Work out the finished part from the listing and answer in its coordinate system (mm). Face numbers are marked on the shaded views. A direction names the side the tool comes from. Coordinates: 2 decimals unless noted, no trailing zeros. Loops run counter-clockwise (first coordinate to the right, second up) from the corner with the lowest first, then second, coordinate; pieces in that order, holes last. Notation, with made-up numbers: (38.25, 76.25) -> (59.25, 76.25) arc R20 cw to (59.25, 97.25) -> close; hole circle Ø11 at (70.5, -3.75). An arc over 180 degrees is marked (long way). Use a Markdown table: item, result.
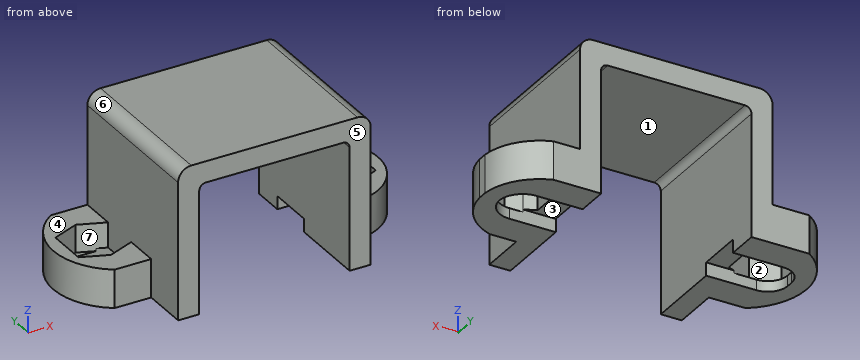
from build123d import *

# Parameters (mm, degrees)
EXTRUDE_1_DEPTH      = 11.4
SKETCH_2_W           = 11.4
SKETCH_2_H           = 8.3
CUT_EXTRUDE_1_DEPTH  = 9.8
CUT_EXTRUDE_2_DEPTH  = 10.6
CUT_EXTRUDE_3_DEPTH  = 0.8
CUT_EXTRUDE_4_DEPTH  = 8.5
CUT_EXTRUDE_5_DEPTH  = 0.8
CUT_EXTRUDE_6_DEPTH  = 2.1
CUT_EXTRUDE_7_DEPTH  = 0.2
CUT_EXTRUDE_8_DEPTH  = 1
CUT_EXTRUDE_9_DEPTH  = 8.5
CUT_EXTRUDE_10_DEPTH = 1.9
CUT_EXTRUDE_11_DEPTH = 0.2
EXTRUDE_2_DEPTH      = 3.5
FILLET_1_R           = 0.5
FILLET_2_R           = 1
FILLET_3_R           = 1.5


with BuildPart() as part:
    # 草图1 → 凸台-拉伸1 (new body)
    with BuildSketch(Plane.XY.offset(1.6)):
        with BuildLine():
            Line((-10.088816953, -2.4), (9.3, -2.4))
            ThreePointArc((9.3, -2.4), (11.373008704, -0.957826085), (12.3, 1.391198782))
            Line((12.3, 1.391198782), (12.3, 2.108801218))
            ThreePointArc((12.3, 2.108801218), (11.373008704, 4.457826085), (9.3, 5.9))
            Line((9.3, 5.9), (-10.088816953, 5.9))
            ThreePointArc((-10.088816953, 5.9), (-12.3, 1.75), (-10.088816953, -2.4))
        make_face()
        with BuildLine():
            Line((-7.8, 0), (-10.8, 0))
            Line((-10.8, 0), (-11.007, 0.0828))
            Line((-11.007, 0.0828), (-11.007, 2))
            ThreePointArc((-11.007, 2), (-10.567660172, 3.060660172), (-9.507, 3.5))
            Line((-9.507, 3.5), (-8.05, 3.5))
            Line((-8.05, 3.5), (-7.3, 3.2))
            Line((-7.3, 3.2), (-7.3, 0.2))
            Line((-7.3, 0.2), (-7.8, 0))
        make_face(mode=Mode.SUBTRACT)
        with BuildLine():
            Line((7.3, 0.4), (7.3, 3.1))
            Line((7.3, 3.1), (8.188888889, 3.5))
            Line((8.188888889, 3.5), (9.206872393, 3.5))
            ThreePointArc((9.206872393, 3.5), (10.461862433, 2.99034879), (11.006177815, 1.75))
            ThreePointArc((11.006177815, 1.75), (10.461862433, 0.50965121), (9.206872393, 0))
            Line((9.206872393, 0), (8.188888889, 0))
            Line((8.188888889, 0), (7.3, 0.4))
        make_face(mode=Mode.SUBTRACT)
    extrude(amount=-EXTRUDE_1_DEPTH)

    # 草图2 → 切除-拉伸1 (cut)
    with BuildSketch(Plane(origin=(0, 0, -9.8), x_dir=(-1, 0, 0), z_dir=(0, 0, -1))):
        with Locations((0, 1.75)):
            Rectangle(SKETCH_2_W, SKETCH_2_H)
    extrude(amount=-CUT_EXTRUDE_1_DEPTH, mode=Mode.SUBTRACT)

    # 草图3 → 切除-拉伸2 (cut)
    with BuildSketch(Plane.XY.offset(1.6)):
        Polygon((-7.8, 0), (-10.8, 0), (-9.3, -0.6), align=None)
    extrude(amount=-CUT_EXTRUDE_2_DEPTH, mode=Mode.SUBTRACT)

    # 草图4 → 切除-拉伸3 (cut)
    with BuildSketch(Plane(origin=(0, 0, -9.8), x_dir=(-1, 0, 0), z_dir=(0, 0, -1))):
        Polygon((11.007, 0.0828), (10.8, 0), (11.007, 0), align=None)
    extrude(amount=-CUT_EXTRUDE_3_DEPTH, mode=Mode.SUBTRACT)

    # 草图5 → 切除-拉伸4 (cut)
    with BuildSketch(Plane.XY.offset(1.6)):
        with BuildLine():
            Line((-9.507, 3.5), (-8.05, 3.5))
            Line((-8.05, 3.5), (-7.3, 3.2))
            Line((-7.3, 3.2), (-7.3, 5.9))
            Line((-7.3, 5.9), (-10.088816953, 5.9))
            ThreePointArc((-10.088816953, 5.9), (-12.3, 1.75), (-10.088816953, -2.4))
            Line((-10.088816953, -2.4), (-7.3, -2.4))
            Line((-7.3, -2.4), (-7.3, 0.2))
            Line((-7.3, 0.2), (-9.3, -0.6))
            Line((-9.3, -0.6), (-11.007, 0.0828))
            Line((-11.007, 0.0828), (-11.007, 2))
            ThreePointArc((-11.007, 2), (-10.567660172, 3.060660172), (-9.507, 3.5))
        make_face()
    extrude(amount=-CUT_EXTRUDE_4_DEPTH, mode=Mode.SUBTRACT)

    # 草图6 → 切除-拉伸5 (cut)
    with BuildSketch(Plane(origin=(0, 0, -9.8), x_dir=(-1, 0, 0), z_dir=(0, 0, -1))):
        Polygon((7.3, 3.2), (8.05, 3.5), (5.7, 3.5), (5.7, 0), (7.8, 0), (7.3, 0.2), align=None)
    extrude(amount=-CUT_EXTRUDE_5_DEPTH, mode=Mode.SUBTRACT)

    # 草图7 → 切除-拉伸6 (cut)
    with BuildSketch(Plane.XY.offset(-6.9)):
        with BuildLine():
            Line((-9.507, 3.5), (-8.05, 3.5))
            Line((-8.05, 3.5), (-9.3, 4))
            Line((-9.3, 4), (-11.3, 3.2))
            Line((-11.3, 3.2), (-11.3, 0.2))
            Line((-11.3, 0.2), (-11.007, 0.0828))
            Line((-11.007, 0.0828), (-11.007, 2))
            ThreePointArc((-11.007, 2), (-10.567660172, 3.060660172), (-9.507, 3.5))
        make_face()
    extrude(amount=-CUT_EXTRUDE_6_DEPTH, mode=Mode.SUBTRACT)

    # 草图8 → 切除-拉伸7 (cut)
    with BuildSketch(Plane(origin=(0, 0, -9), x_dir=(-1, 0, 0), z_dir=(0, 0, -1))):
        Polygon((7.3, 3.2), (8.05, 3.5), (5.7, 3.5), (5.7, 0), (7.8, 0), (7.3, 0.2), align=None)
    extrude(amount=-CUT_EXTRUDE_7_DEPTH, mode=Mode.SUBTRACT)

    # 草图9 → 切除-拉伸8 (cut)
    with BuildSketch(Plane(origin=(0, 0, -9.8), x_dir=(-1, 0, 0), z_dir=(0, 0, -1))):
        Polygon((-7.3, 0.4), (-8.188888889, 0), (-5.7, 0), (-5.7, 3.5), (-8.188888889, 3.5), (-7.3, 3.1), align=None)
    extrude(amount=-CUT_EXTRUDE_8_DEPTH, mode=Mode.SUBTRACT)

    # 草图10 → 切除-拉伸9 (cut)
    with BuildSketch(Plane.XY.offset(1.6)):
        with BuildLine():
            Line((9.206872393, 0), (8.188888889, 0))
            Line((8.188888889, 0), (7.3, 0.4))
            Line((7.3, 0.4), (7.3, -2.4))
            Line((7.3, -2.4), (9.3, -2.4))
            ThreePointArc((9.3, -2.4), (11.373008704, -0.957826085), (12.3, 1.391198782))
            Line((12.3, 1.391198782), (12.3, 2.108801218))
            ThreePointArc((12.3, 2.108801218), (11.373008704, 4.457826085), (9.3, 5.9))
            Line((9.3, 5.9), (7.3, 5.9))
            Line((7.3, 5.9), (7.3, 3.1))
            Line((7.3, 3.1), (8.188888889, 3.5))
            Line((8.188888889, 3.5), (9.206872393, 3.5))
            ThreePointArc((9.206872393, 3.5), (10.461862433, 2.99034879), (11.006177815, 1.75))
            ThreePointArc((11.006177815, 1.75), (10.461862433, 0.50965121), (9.206872393, 0))
        make_face()
    extrude(amount=-CUT_EXTRUDE_9_DEPTH, mode=Mode.SUBTRACT)

    # 草图11 → 切除-拉伸10 (cut)
    with BuildSketch(Plane.XY.offset(-6.9)):
        with BuildLine():
            Line((9.206872393, 0), (8.188888889, 0))
            Line((8.188888889, 0), (9.3, -0.5))
            Line((9.3, -0.5), (11.3, 0.3))
            Line((11.3, 0.3), (11.3, 3.2))
            Line((11.3, 3.2), (9.3, 4))
            Line((9.3, 4), (8.188888889, 3.5))
            Line((8.188888889, 3.5), (9.206872393, 3.5))
            ThreePointArc((9.206872393, 3.5), (10.461862433, 2.99034879), (11.006177815, 1.75))
            ThreePointArc((11.006177815, 1.75), (10.461862433, 0.50965121), (9.206872393, 0))
        make_face()
    extrude(amount=-CUT_EXTRUDE_10_DEPTH, mode=Mode.SUBTRACT)

    # 草图12 → 切除-拉伸11 (cut)
    with BuildSketch(Plane.XY.offset(-8.8)):
        with BuildLine():
            Line((9.206872393, 0), (8.188888889, 0))
            Line((8.188888889, 0), (9.3, -0.5))
            Line((9.3, -0.5), (11.3, 0.3))
            Line((11.3, 0.3), (11.3, 3.2))
            Line((11.3, 3.2), (9.3, 4))
            Line((9.3, 4), (8.188888889, 3.5))
            Line((8.188888889, 3.5), (9.206872393, 3.5))
            ThreePointArc((9.206872393, 3.5), (10.461862433, 2.99034879), (11.006177815, 1.75))
            ThreePointArc((11.006177815, 1.75), (10.461862433, 0.50965121), (9.206872393, 0))
        make_face()
    extrude(amount=-CUT_EXTRUDE_11_DEPTH, mode=Mode.SUBTRACT)

    # 草图13 → 凸台-拉伸2 (add)
    with BuildSketch(Plane.XZ.offset(2.4)):
        Polygon((-7.3, 1.6), (7.3, 1.6), (7.3, -9.8), (5.7, -9.8), (5.7, 0), (-5.7, 0), (-5.7, -9.8), (-7.3, -9.8), align=None)
    extrude(amount=EXTRUDE_2_DEPTH)

    # 圆角1
    fillet_1_edges = [part.edges().sort_by_distance(p)[0] for p in [
        (5.7, 0, 0),
        (-5.7, 0, 0),
    ]]
    fillet(fillet_1_edges, radius=FILLET_1_R)

    # 圆角2
    fillet_2_edges = [part.edges().sort_by_distance(p)[0] for p in [
        (-7.3, 0, 1.6),
        (7.3, 0, 1.6),
    ]]
    fillet(fillet_2_edges, radius=FILLET_2_R)

    # 圆角3
    # the kernel refuses this fillet: 1.5 mm, written as the material it adds along each edge
    with BuildSketch(Plane(origin=(-11.007, 0, -9.8), x_dir=(1.0, 7.597747752272154e-12, 0), z_dir=(0, 0, 1))) as fillet_3_piece_1:
        with BuildLine():
            CenterArc((FILLET_3_R, FILLET_3_R), FILLET_3_R, 180, 90)
            Line((0, FILLET_3_R), (0, 0))
            Line((0, 0), (FILLET_3_R, 0))
        make_face()
    extrude(amount=0.8)


solid = part.part
Q1. Section B-B on x = 7.75 is taken. Determine the outline of the cut face in (y, z), and give its area (3 significant figures).
Solved:
| item | result |
|---|---|
| outline | (-2.4, -9.8) -> (0, -9.8) -> (0, -8.8) -> (0.2, -8.8) -> (0.2, -6.9) -> (-2.4, -6.9) -> close; (3.3, -8.8) -> (3.5, -8.8) -> (3.5, -9.8) -> (5.9, -9.8) -> (5.9, -6.9) -> (3.3, -6.9) -> close |
| area | 14.7 mm² |
Q2. Section C-C on y = -4.75 is taken. Determine the outline of the cut face in (x, z).
Solved:
| item | result |
|---|---|
| outline | (-7.3, -9.8) -> (-5.7, -9.8) -> (-5.7, -0.5) arc R0.5 cw to (-5.2, 0) -> (5.2, 0) arc R0.5 cw to (5.7, -0.5) -> (5.7, -9.8) -> (7.3, -9.8) -> (7.3, 0.6) arc R1 ccw to (6.3, 1.6) -> (-6.3, 1.6) arc R1 ccw to (-7.3, 0.6) -> close |
Q3. Section D-D on y = 0.75 is taken. Determine the outline of the cut face in (x, z).
Solved:
| item | result |
|---|---|
| outline | (-12.2, -9.8) -> (-10.81, -9.8) -> (-10.81, -9) -> (-11.3, -9) -> (-11.3, -6.9) -> (-12.2, -6.9) -> close; (-7.3, -8.8) -> (-5.7, -8.8) -> (-5.7, -0.5) arc R0.5 cw to (-5.2, 0) -> (5.2, 0) arc R0.5 cw to (5.7, -0.5) -> (5.7, -8.8) -> (7.3, -8.8) -> (7.3, 0.6) arc R1 ccw to (6.3, 1.6) -> (-6.3, 1.6) arc R1 ccw to (-7.3, 0.6) -> close; (10.67, -9.8) -> (12.2, -9.8) -> (12.2, -6.9) -> (11.3, -6.9) -> (11.3, -9) -> (10.67, -9) -> close |
Q4. Determine the mould class of the marked faces 5, 6 and 7 for opening direction Y: pulls with the +Y half, pulls with the -Y half, needs draft (parallel to the pull), parting line crosses it, or undercut.
Solved:
| item | result |
|---|---|
| face 5 | pulls with the -Y half |
| face 6 | needs draft |
| face 7 | undercut |
Q5. For the marked faces 1, 2, 3 and 4, determine the directions among +Z, -Z, +X, -X, +Y, -Y from which every point of the face is accessible in a straight line to the end or side of a thin tool.
Solved:
| item | result |
|---|---|
| face 1 | -Z, +Y, -Y |
| face 2 | +Z |
| face 3 | -Z |
| face 4 | +Z, -X, +Y, -Y |
Q6. Section A-A on z = -2.5 is taken. Determine the outline of the cut face in (x, y).
Solved:
| item | result |
|---|---|
| outline | (-7.3, -5.9) -> (-5.7, -5.9) -> (-5.7, 5.9) -> (-7.3, 5.9) -> close; (5.7, -5.9) -> (7.3, -5.9) -> (7.3, 5.9) -> (5.7, 5.9) -> close |
Q7. Consider line 1 (X direction, y = -4.25, z = -2.5); line 2 (Z direction, x = -3.5, y = -3); line 3 (X direction, y = 3, z = -8.25). Determine where each line is inside the solid, lowest interval first. Write a range as [from, to].
Solved:
| item | result |
|---|---|
| line 1 | [-7.3, -5.7], [5.7, 7.3] |
| line 2 | [0, 1.6] |
| line 3 | [-12.14, -11.3], [-7.3, -5.7], [5.7, 7.3], [11.3, 12.13] |
Q8. Given pin 1 Ø5 at (y, z) = (3.5, -4.5) entering from -X; pin 2 Ø4 at (x, y) = (9.5, 0.5) entering from +Z; pin 3 Ø3 at (y, z) = (-1, -6.5) entering from +X, each flat-ended and moving along its own axis, determine where each tip first touches the part or whether it passes through.
Solved:
| item | result |
|---|---|
| pin 1 | x = -12.19 |
| pin 2 | z = -6.9 |
| pin 3 | x = 12.12 |
